Autodesk Inventor part; units mm, degrees
ref_plane "YZ Plane" through (0, 0, 0) normal (1, 0, 0) x (0, 1, 0)
ref_plane "XZ Plane" through (0, 0, 0) normal (0, 1, 0) x (-1, 0, 0)
ref_plane "XY Plane" through (0, 0, 0) normal (0, 0, 1) x (1, 0, 0)
sketch "Sketch1" plane through (0, 0, 0) normal (0, 1, 0) x (-1, 0, 0)
  line L0 (0, 0) -> (93, 0)
  line L1 (93, 0) -> (93, -90)
  line L2 (93, -90) -> (0, -90)
  line L3 (0, -90) -> (0, 0)
  line L4 (95, -92) -> (95, 2)
  line L5 (95, 2) -> (-2, 2)
  line L6 (-2, 2) -> (-2, -92)
  line L7 (-2, -92) -> (95, -92)
  line L8 (85.55, -11.63) -> (7.45, -11.63)
  line L9 (7.45, -11.63) -> (7.45, -62.73)
  line L10 (7.45, -62.73) -> (85.55, -62.73)
  line L11 (85.55, -62.73) -> (85.55, -11.63)
  line L12 (82.5, -17.18) -> (10.5, -17.18)
  line L13 (10.5, -17.18) -> (10.5, -57.18)
  line L14 (10.5, -57.18) -> (82.5, -57.18)
  line L15 (82.5, -57.18) -> (82.5, -17.18)
  arc A0 (90.8, 0) -> (93, -8.4256) centre (90.8, -4.5) ccw
  arc A1 (0, -8.4256) -> (2.2, 0) centre (2.2, -4.5) ccw
  arc A2 (93, -66.31) -> (93, -75.29) centre (90.8, -70.8) ccw
  arc A3 (0, -75.29) -> (0, -66.31) centre (2.2, -70.8) ccw
  point P0 (10.5, -37.18)
  point P1 (7.45, -37.18)
  point P2 (46.5, -62.73)
  point P3 (46.5, -57.18)
  dimension "d0" = 93
  dimension "d1" = 90
  dimension "d2" = 2
  dimension "d7" = 78.1
  dimension "d8" = 51.1
  dimension "d9" = 72
  dimension "d10" = 40
extrude "Extrusion1" add sketch "Sketch1" along normal blind 2 contours L0 A0 L1 A2 L2 L3 A3 A1
extrude "Extrusion2" add sketch "Sketch1" along normal blind 10.5 contours L0 A1 L3 | L0 L1 A0 | A3 L3 | L1 A2
extrude "Extrusion3" add sketch "Sketch1" along normal blind 17.5 contours L7 L6 L5 L4
chamfer "Chamfer1" distance 2 angle 45 4 edges at (-46.5, 0, -11.63) (-85.55, 0, -37.18) (-7.45, 0, -37.18) (-46.5, 0, -62.73)
fillet "Fillet1" radius 2 8 edges at (-46.5, 0, -92) (2, 0, -45) (2, 8.75, -92) (-95, 8.75, -92) (-95, 0, -45) (-46.5, 0, 2) (-95, 8.75, 2) (2, 8.75, 2)
sketch "Sketch2" plane through (0, 10.5, 0) normal (0, 1, 0) x (1, 0, 0)
  circle A0 centre (-90.8, 4.5) radius 1.15
  circle A1 centre (-90.8, 70.8) radius 1.15
  circle A2 centre (-2.2, 70.8) radius 1.15
  circle A3 centre (-2.2, 4.5) radius 1.15
  point P0 (0, 0)
  dimension "d26" = 2.3
  dimension "d27" = 2.3
  dimension "d28" = 2.3
  dimension "d29" = 2.3
extrude "Extrusion4" cut sketch "Sketch2" against normal blind 7
sketch "Sketch3" plane through (0, 17.5, 0) normal (0, 1, 0) x (1, 0, 0)
  circle A0 centre (-2.2, 4.5) radius 1.15
  circle A1 centre (-90.8, 4.5) radius 1.15
  circle A2 centre (-90.8, 70.8) radius 1.15
  circle A3 centre (-2.2, 70.8) radius 1.15
  circle A4 centre (-90.8, 70.8) radius 3.125
  circle A5 centre (-90.8, 4.5) radius 3.125
  circle A6 centre (-2.2, 4.5) radius 3.125
  circle A7 centre (-2.2, 70.8) radius 3.125
  point P0 (0, 0)
  dimension "d32" = 6.25
  dimension "d33" = 6.25
  dimension "d34" = 6.25
  dimension "d35" = 6.25
extrude "Extrusion5" cut sketch "Sketch3" against normal blind 3 contours A0 | A1 | A2 | A3 | A4 | A5 | A6 | A7
properties part number "caseFront"
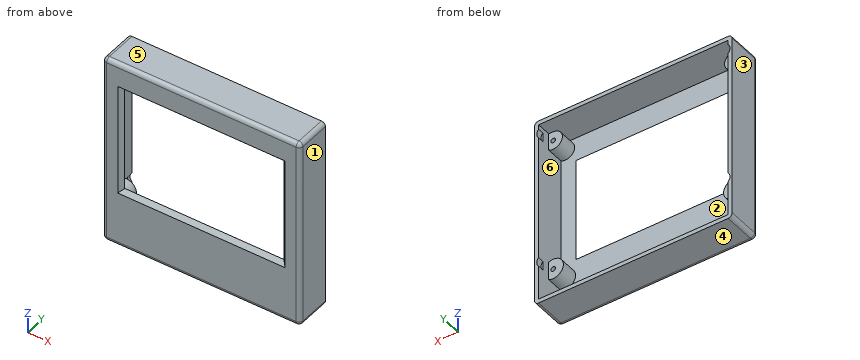
Geometry: final body of the model. Coordinates: model frame, mm. Face numbers are marked on the shaded views. A direction names the side the tool comes from. Give positions to 0.01 mm unless a question says otherwise; leave off trailing zeros. Write each loop counter-clockwise with the first axis right and the second up, starting at its lowest first coordinate (ties: lowest second). Pieces come first, ordered by that corner, then holes. Notation, with made-up numbers: M 46,56 L 67,56 A18 cw 67,69 Z; hole C -36,-15 d3. An arc over 180 degrees is marked long. Answer in a Markdown table with one row per item. Add a question column.
(1) First-contact query: pin 1 (0.5 mm diameter, centred on x = 0.5, z = -70.5, fed in from +Y); pin 2 (2 mm diameter, centred on x = -4.5, z = -4, fed in from +Y); pin 3 (10 mm diameter, centred on x = -82.5, z = -29, fed in from +Y). Flat tips, straight axial feed; report the tip coordinate or a pass-through.
(2) Reachability of the marked faces 1 and 2 from +Z, -Z, +X, -X, +Y, -Y: full face, straight path, thin tool, end or side. Return the list, or none.
(3) Section C-C on z = -4.5. Return loops of the section in (x, y) (3 decimals), and give its area (3 significant figures).
(4) Ray query, line 1 (Z direction, x = -53.5, y = 7); line 2 (X direction, y = 3.75, z = -49); line 3 (Z direction, x = -5, y = 7.5). Return the intervals inside material, ascending.
(5) Mould query, pull axis Z, two halves, no side actions, for the marked faces 3, 4, 5 and 6. Classes: +Z half, -Z half, draft (parallel to the pull), parting line (faces both ways), or undercut.
(6) Section D-D on z = -70.8. Return loops of the section in (x, y) (3 decimals).
Result set:
| question | item | result |
|---|---|---|
| 1 | pin 1 | stops at y = 14.5 |
| 1 | pin 2 | stops at y = 10.5 |
| 1 | pin 3 | stops at y = 2 |
| 2 | face 1 | +Z, -Z, +X, +Y, -Y |
| 2 | face 2 | +Y |
| 3 | outline | M -95,2 A2 ccw -93,0 L 0,0 A2 ccw 2,2 L 2,17.5 L 0.925,17.5 L 0.925,14.5 L 0,14.5 L 0,10.5 L -1.05,10.5 L -1.05,3.5 L -3.35,3.5 L -3.35,10.5 L -6.7,10.5 L -6.7,2 L -86.3,2 L -86.3,10.5 L -89.65,10.5 L -89.65,3.5 L -91.95,3.5 L -91.95,10.5 L -93,10.5 L -93,14.5 L -93.925,14.5 L -93.925,17.5 L -95,17.5 Z |
| 3 | area | 330 mm^2 |
| 4 | line 1 | z = -92 to -90, 0 to 2 |
| 4 | line 2 | x = -95 to -93, 0 to 2 |
| 4 | line 3 | z = -92 to -90, -74.94 to -66.66, -8.02 to -0.98, 0 to 2 |
| 5 | face 3 | draft |
| 5 | face 4 | -Z half |
| 5 | face 5 | +Z half |
| 5 | face 6 | undercut |
| 6 | outline | M -95,2 A2 ccw -93,0 L 0,0 A2 ccw 2,2 L 2,17.5 L 0.925,17.5 L 0.925,14.5 L 0,14.5 L 0,10.5 L -1.05,10.5 L -1.05,3.5 L -3.35,3.5 L -3.35,10.5 L -7.2,10.5 L -7.2,2 L -85.8,2 L -85.8,10.5 L -89.65,10.5 L -89.65,3.5 L -91.95,3.5 L -91.95,10.5 L -93,10.5 L -93,14.5 L -93.925,14.5 L -93.925,17.5 L -95,17.5 Z |
